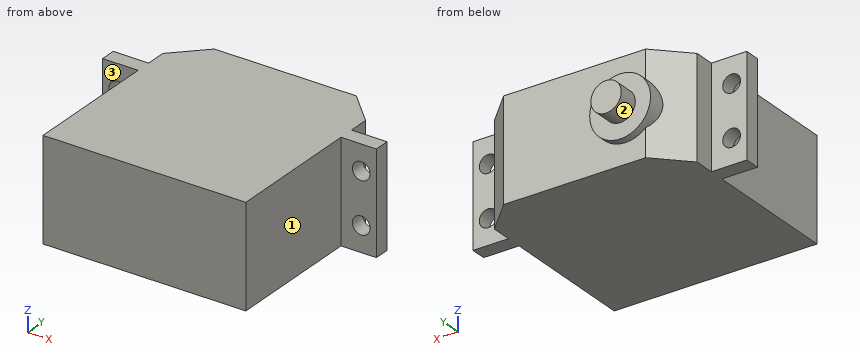
from build123d import *

# Parameters (mm, degrees)
SKETCH_1_W           = 40
SKETCH_1_H           = 40
EXTRUDE_1_DEPTH      = 10
SKETCH_2_W           = 54
SKETCH_2_H           = 3
EXTRUDE_2_DEPTH      = 10
CHAMFER_1_SIZE       = 6
EXTRUDE_3_DEPTH      = 1.5
EXTRUDE_3_DEPTH_BACK = 20
SKETCH_4_R           = 6
SKETCH_5_R           = 3
EXTRUDE_4_DEPTH      = 4
SKETCH_6_R           = 1.75
CUT_EXTRUDE_1_DEPTH  = 57.648036153


with BuildPart() as part:
    # 草图1 → 凸台-拉伸1 (new, symmetric)
    with BuildSketch(Plane.XY):
        with Locations((20, 20)):
            Rectangle(SKETCH_1_W, SKETCH_1_H)
    extrude(amount=EXTRUDE_1_DEPTH, both=True)

    # 草图2 → 凸台-拉伸2 (add, symmetric)
    with BuildSketch(Plane.XY):
        with Locations((20, 28.5)):
            Rectangle(SKETCH_2_W, SKETCH_2_H)
    extrude(amount=EXTRUDE_2_DEPTH, both=True)

    # 倒角1
    chamfer_1_edges = [part.edges().sort_by_distance(p)[0] for p in [
        (0, 40, 0),
        (40, 40, 0),
    ]]
    chamfer(chamfer_1_edges, length=CHAMFER_1_SIZE)

    # 草图4 → 凸台-拉伸3 (add, two sides: drawn at the far end of the back side and taken through both)
    with BuildSketch(Plane(origin=(0, 40, 0), x_dir=(1, 0, 0), z_dir=(0, 1, 0)).offset(-EXTRUDE_3_DEPTH_BACK)):
        with Locations(Location((10, 0, 0), (0, 0, 270))):
            Circle(SKETCH_4_R)
    extrude(amount=EXTRUDE_3_DEPTH + EXTRUDE_3_DEPTH_BACK)

    # 草图5 → 凸台-拉伸4 (add)
    with BuildSketch(Plane(origin=(0, 41.5, 0), x_dir=(1, 0, 0), z_dir=(0, 1, 0))):
        with Locations(Location((10, 0, 0), (0, 0, 270))):
            Circle(SKETCH_5_R)
    extrude(amount=EXTRUDE_4_DEPTH)

    # 草图6 → 切除-拉伸1 (cut, through all)
    with BuildSketch(Plane(origin=(0, 30, 0), x_dir=(1, 0, 0), z_dir=(0, 1, 0))):
        with Locations(Location((-4, 5, 0), (0, 0, 270))):
            Circle(SKETCH_6_R)
        with Locations(Location((-4, -5, 0), (0, 0, 270))):
            Circle(SKETCH_6_R)
        with Locations(Location((44, 5, 0), (0, 0, 270))):
            Circle(SKETCH_6_R)
        with Locations(Location((44, -5, 0), (0, 0, 270))):
            Circle(SKETCH_6_R)
    extrude(amount=-CUT_EXTRUDE_1_DEPTH, mode=Mode.SUBTRACT)


solid = part.part
Work out the finished part from the listing and answer in its coordinate system (mm). Face numbers are marked on the shaded views. A direction names the side the tool comes from. Round coordinates to 2 decimals unless told otherwise and drop trailing zeros. Loops run counter-clockwise (first coordinate to the right, second up) from the corner with the lowest first, then second, coordinate; pieces in that order, holes last. Notation, with made-up numbers: (-30, 36) -> (-25, 36) arc R10 ccw to (-25, 40) -> close; hole circle Ø4 at (-25, 59.5). An arc over 180 degrees is marked (long way). Use one line per item in the form item = value.
(1) Find section D-D on z = -1.75. Give the vertices of the cut face in (x, y), then the cut area to 3 significant figures.
Answer list:
outline = (-7, 27) -> (0, 27) -> (0, 0) -> (40, 0) -> (40, 27) -> (47, 27) -> (47, 30) -> (40, 30) -> (40, 34) -> (34, 40) -> (15.74, 40) -> (15.74, 41.5) -> (12.44, 41.5) -> (12.44, 45.5) -> (7.56, 45.5) -> (7.56, 41.5) -> (4.26, 41.5) -> (4.26, 38.26) -> (0, 34) -> (0, 30) -> (-7, 30) -> close
area = 1,640 mm2
(2) Find section C-C on x = 10. Give the vertices of the cut face in (y, z), then the cut area to 3 significant figures.
Answer list:
outline = (0, -10) -> (40, -10) -> (40, -6) -> (41.5, -6) -> (41.5, -3) -> (45.5, -3) -> (45.5, 3) -> (41.5, 3) -> (41.5, 6) -> (40, 6) -> (40, 10) -> (0, 10) -> close
area = 842 mm2
(3) Flat-ended cylindrical pins translate along their axes: P1, Ø8, axis at y = 15, z = 3.5, coming from the +X side; P2, Ø4.5, axis at y = 33, z = 2, coming from the -X side; P3, Ø4, axis at x = -4, z = -5, coming from the -Y side; P4, Ø10, axis at y = 30.5, z = 0.5, coming from the +X side. Find the tip coordinate at first contact, or state that the pin passes through.
Answer list:
P1 = 40
P2 = 0
P3 = 27
P4 = 47
(4) A tool of negligible diameter and unlimited length cuts with its end or side. For the marked faces 1, 2 and 3, from which of +Z, -Z, +X, -X, +Y, -Y can it reach the whole face along a straight path? Write none if from no direction.
Answer list:
face_1 = +Z, -Z, +X, -Y
face_2 = +Y
face_3 = +Z, -Z, -X, -Y
(5) Find section B-B on y = 29. Give the vertices of the cut face in (x, z).
Answer list:
outline = (-7, -10) -> (47, -10) -> (47, 10) -> (-7, 10) -> close; hole circle Ø3.5 at (-4, -5); hole circle Ø3.5 at (-4, 5); hole circle Ø3.5 at (44, -5); hole circle Ø3.5 at (44, 5)
(6) Find section A-A on x = -4. Give the vertices of the cut face in (y, z), then the cut area to 3 significant figures.
Answer list:
outline = (27, -10) -> (30, -10) -> (30, -6.75) -> (27, -6.75) -> close; (27, -3.25) -> (30, -3.25) -> (30, 3.25) -> (27, 3.25) -> close; (27, 6.75) -> (30, 6.75) -> (30, 10) -> (27, 10) -> close
area = 39.0 mm2
(7) Straight lines are drawn through the part: line 1 (X direction, y = 28.7, z = -5); line 2 (Y direction, x = 6, z = -5.5); line 3 (Y direction, x = 41, z = 5.25). For each, find the intervals that lie inside material, in ascending order.
Answer list:
line_1 = -7 to -5.75, -2.25 to 42.25, 45.75 to 47
line_2 = 0 to 40
line_3 = 27 to 30
